Input: part model. Units: mm. Frame: model coordinates. A direction names the side the tool comes from. Coordinates: 2 decimals unless noted, no trailing zeros. Order: outer loops, then holes, each group sorted by start corner. A loop starts at its lowest first (then second) coordinate and runs counter-clockwise, first axis right, second up. Notation, with made-up numbers: (33, -31) - (53, -31) arc R19 ccw to (53, -19) - close; hole circle Ø6 at (-4, 42). An arc over 180 degrees is marked (long way). Answer as CSV lines item,"result". Start each with the question number.
Item 1: Section A-A (x = 0). Output: boundary loops of the cut face in (y, z).
Item 2: Material intervals for line 1 along Z through (x, y) = (0, 1.4); line 2 along Z through (x, y) = (6, -0.3); line 3 along X through (y, z) = (0.75, 5.75), sorted ascending.
Item 3: Draft query along Z for faces 1 (the flat face through (0, 2, -2.333)), 2 (the flat face through (0, -1.25, 6)), 3 (the cylindrical face through (-0.273, 2.465, 0.585)). Return one class per face: +Z half, -Z half, draft (parallel to the pull), parting line (faces both ways), or undercut.
Item 4: Access query for faces 4 (the flat face through (-0.1, 1.25, 6.5)), 5 (the flat face through (-7, 0, 1.667)), 6 (the flat face through (-3.053, 3.099, 4.671)), 7 (the flat face through (8, 0, 1.667)), 8 (the flat face through (0, 3, 6.021)). Directions: +Z, -Z, +X, -X, +Y, -Y. A direction counts if a zero-diameter tool reaches every point of the face in a straight line with its end or side. Return the directions, or none.
Item 5: Section B-B (y = 2.25). Output: boundary loops of the cut face in (x, z), and give its area (3 significant figures).
Item 6: First-contact query: pin 1 (2 mm diameter, centred on y = 3, z = 0, fed in from -X); pin 2 (0.8 mm diameter, centred on x = 6.5, y = -0.5, fed in from -Z); pin 3 (1 mm diameter, centred on y = 2.5, z = 3, fed in from +X); pin 4 (3 mm diameter, centred on x = 6, z = 5.67, fed in from +Y). Flat tips, straight axial feed; report the tip coordinate or a pass-through.
Item 7: Section C-C (z = 6.25). Output: boundary loops of the cut face in (x, y), and give its area (3 significant figures).
Item 8: Section D-D (z = 1.25). Output: boundary loops of the cut face in (x, y).
from build123d import *

# Parameters (mm, degrees)
SKETCH1_R           = 1.6
SKETCH1_R_2         = 2.5
BOSS_EXTRUDE1_DEPTH = 1.25
SKETCH2_R           = 2.1
BOSS_EXTRUDE2_DEPTH = 5


with BuildPart() as part:
    # Sketch1 → Boss-Extrude1 (new body, symmetric)
    with BuildSketch(Plane(origin=(0, 0, 0), x_dir=(1, 0, 0), z_dir=(0, 1, 0))):
        Polygon((-5, -1.666666667), (-10, -1.666666667), (-10, -9.666666667), (10, -9.666666667), (10, -1.666666667), (5, -1.666666667), (5, 2.333333333), (-5, 2.333333333), align=None)
        with Locations((-6, -5.666666667)):
            Circle(SKETCH1_R, mode=Mode.SUBTRACT)
        with Locations((6, -5.666666667)):
            Circle(SKETCH1_R, mode=Mode.SUBTRACT)
        with Locations((0, -2.666666667)):
            Circle(SKETCH1_R_2, mode=Mode.SUBTRACT)
    extrude(amount=BOSS_EXTRUDE1_DEPTH, both=True)

    # Sketch2 → Boss-Extrude2 (add)
    with BuildSketch(Plane(origin=(0, 0, 0), x_dir=(1, 0, 0), z_dir=(0, 1, 0))):
        Polygon((-5, 2.333333333), (-5, -1.666666667), (-4.260765506, -3.357761167), (-1.81082534, -6.020739609), (1.81082534, -6.020739609), (4.260765506, -3.357761167), (5, -1.666666667), (5, 2.333333333), align=None)
        with Locations((0, -2.666666667)):
            Circle(SKETCH2_R, mode=Mode.SUBTRACT)
    extrude(amount=BOSS_EXTRUDE2_DEPTH)


solid = part.part
Determined:
1,outline,"(-1.25, -2.33) - (5, -2.33) - (5, 0.57) - (0, 0.57) - (0, 0.17) - (-1.25, 0.17) - close; (-1.25, 5.17) - (0, 5.17) - (0, 4.77) - (5, 4.77) - (5, 6.02) - (1.25, 6.02) - (1.25, 9.67) - (-1.25, 9.67) - close"
2,line 1,"z = -2.33 to 0.57, 4.77 to 6.02"
2,line 2,"z = 1.67 to 4.07, 7.27 to 9.67"
2,line 3,"x = -10 to -7.6, -4.4 to 4.4, 7.6 to 10"
3,face 1,"-Z half"
3,face 2,"draft"
3,face 3,"undercut"
4,face 4,"+Z, +Y"
4,face 5,"-Z, -X, +Y, -Y"
4,face 6,"+Z, -X, +Y"
4,face 7,"-Z, +X, +Y, -Y"
4,face 8,"+Z, +X, -X, +Y"
5,outline,"(-5, -2.33) - (5, -2.33) - (5, 1.67) - (4.26, 3.36) - (1.81, 6.02) - (-1.81, 6.02) - (-4.26, 3.36) - (-5, 1.67) - close; hole circle Ø4.2 at (0, 2.67)"
5,area,"58.0 mm^2"
6,pin 1,"stops at x = -5"
6,pin 2,"stops at z = 1.67"
6,pin 3,"stops at x = 4.64"
6,pin 4,"passes through"
7,outline,"(-10, -1.25) - (-7.49, -1.25) - (-7.49, 1.25) - (-10, 1.25) - close; (-4.51, -1.25) - (4.51, -1.25) - (4.51, 1.25) - (-4.51, 1.25) - close; (7.49, -1.25) - (10, -1.25) - (10, 1.25) - (7.49, 1.25) - close"
7,area,"35.1 mm^2"
8,outline,"(-5, -1.25) - (-2.06, -1.25) - (-2.06, 0) - (-1.55, 0) - (-1.55, 5) - (-5, 5) - close; (1.55, 0) - (2.06, 0) - (2.06, -1.25) - (5, -1.25) - (5, 5) - (1.55, 5) - close"
